Can you work these out from the drawing? Everything is in mm from the part's minimum corner. Give positions to 0.01 mm unless a question says otherwise; leave off trailing zeros. Write each loop counter-clockwise with the first axis right and the second up, starting at its lowest first coordinate (ties: lowest second). Pieces come first, ordered by that corner, then holes. Notation, with made-up numbers: (85, -16) -> (113, -16) arc R30 cw to (113, 21) -> close; hole circle Ø5 at (14.25, 13). An arc over 180 degrees is marked (long way). Return JSON: item names as keys, results as strings.
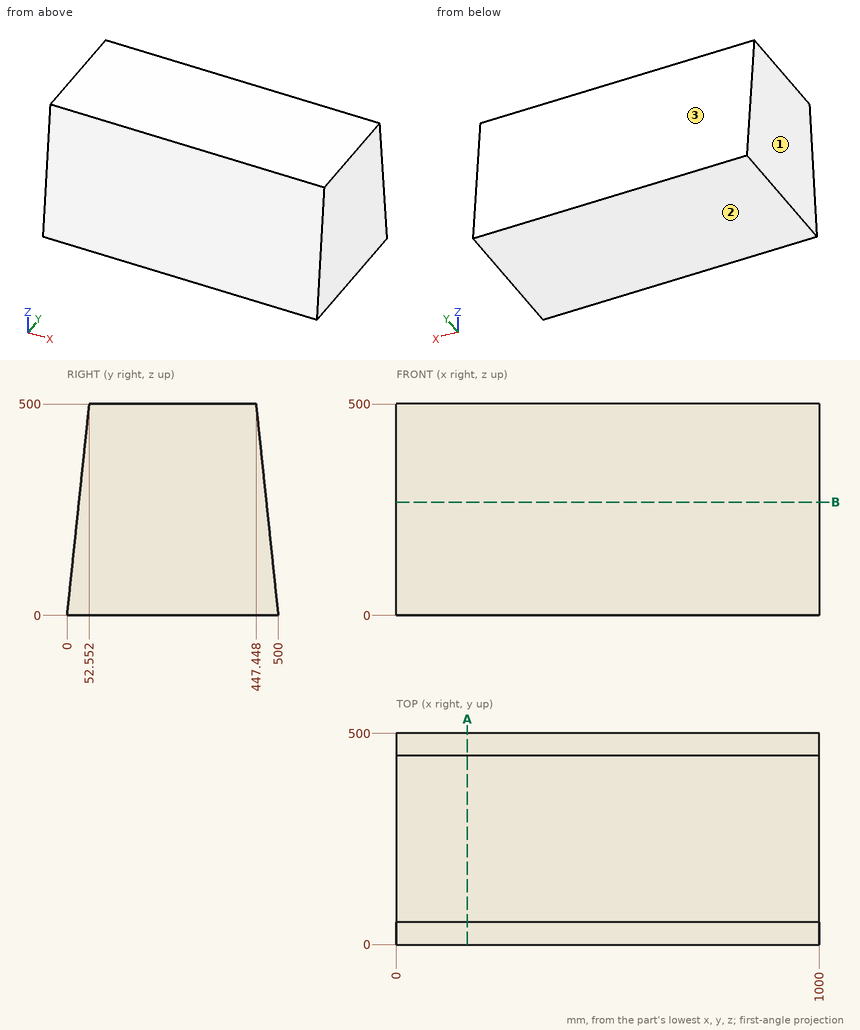
1. Suppose I cut it at A-A, the plane x = 168. List the corners of the cut face in (y, z) for me.
Taken from the geometry:
{"outline": "(0, 0) -> (500, 0) -> (447.45, 500) -> (52.55, 500) -> close"}
2. If I drill on line 1 (Y direction, x = 957, z = 205.5); line 2 (Y direction, x = 732.5, z = 87), over which ranges is the centre line in solid material (lowest first)? Write a range as [from, to].
Taken from the geometry:
{"line 1": "y = [21.6, 478.4]", "line 2": "y = [9.14, 490.86]"}
3. If we mould it in two halves opening along Z, with no side actions, what happens to the marked faces 1, 2 and 3? For each: released by +Z, released by -Z, zero draft, split by the parting line, or undercut.
Taken from the geometry:
{"face 1": "zero draft", "face 2": "released by -Z", "face 3": "released by +Z"}
4. For pin 1 Ø2 at (x, z) = (142, 219) entering from -Y; pin 2 Ø1.5 at (x, z) = (436, 69.5) entering from -Y; pin 3 Ø8 at (x, z) = (422.5, 358.5) entering from -Y, each with a flat end and sliding along its axis, tell me the tip position at first contact or that it passes through.
Taken from the geometry:
{"pin 1": "stops at y = 22.91", "pin 2": "stops at y = 7.23", "pin 3": "stops at y = 37.26"}
5. Suppose I cut it at B-B, the plane z = 268. List the corners of the cut face in (x, y) for me.
Taken from the geometry:
{"outline": "(0, 28.17) -> (1000, 28.17) -> (1000, 471.83) -> (0, 471.83) -> close"}
